Design review of the part built by this model. Coordinates are the model's own, in mm. Face numbers are marked on the shaded views. A direction names the side the tool comes from. Coordinates: 2 decimals unless noted, no trailing zeros. Write each loop counter-clockwise with the first axis right and the second up, starting at its lowest first coordinate (ties: lowest second). Pieces come first, ordered by that corner, then holes.
Q1. Add section B-B, the plane y = 8.25. Give the boundary of the cut face in (x, z), plus the area to 3 significant figures.
Q2. To check wall thickness, follow probe 1 along X at (y, z) = (8.25, 8.75); probe 2 along Y at (x, z) = (16.6, 3); probe 3 along X at (y, z) = (4.25, 10). State the ranges of each line that lie inside material, in increasing order.
Q3. Add section D-D, the plane z = 6. Give the boundary of the cut face in (x, y), plus the area to 3 significant figures.
Q4. The part is to be moulded in two halves that separate along X. For the marked faces 6, 7, 8 and 9, say which applies: +X half, -X half, draft (parallel to the pull), parting line (faces both ways), or undercut.
Q5. Add section A-A, the plane x = 16.6. Give the boundary of the cut face in (y, z).
Q6. Add section C-C, the plane z = 11.5. Give the boundary of the cut face in (x, y), plus the area to 3 significant figures.
Q7. Machinability: for the marked faces 1, 2, 3, 4 and 5, which of the approach directions +Z, -Z, +X, -X, +Y, -Y give a long, thin tool a straight path to every point of the face, cutting with its end or side? Answer none if there is none.
Q8. Clearance check with flat-ended pins moving along their axes: pin 1 Ø2.5 at (x, y) = (31.5, 16) entering from +Z; pin 2 Ø1.7 at (x, z) = (31, 9) entering from -Y; pin 3 Ø6 at (x, y) = (16.6, 6.5) entering from -Z. State where each tip first meets the part, or that it passes through.
from build123d import *

# Parameters (mm, degrees)
EXTRUDE_1_DEPTH     = 3.2
EXTRUDE_2_DEPTH     = 2.6
EXTRUDE_3_DEPTH     = 3
CUT_EXTRUDE_1_DEPTH = 2.1
SKETCH_5_R          = 2.6
CUT_EXTRUDE_2_DEPTH = 1.1
CUT_EXTRUDE_3_DEPTH = 2.1
SKETCH_7_R          = 2.6
CUT_EXTRUDE_4_DEPTH = 0.9
SKETCH_8_R          = 2
CUT_EXTRUDE_5_DEPTH = 1.8


with BuildPart() as part:
    # ｽｹｯﾁ1 → ﾎﾞｽ - 押し出し1 (new body)
    with BuildSketch(Plane.XY):
        with BuildLine():
            Line((0, 0), (13.621587752, 0))
            ThreePointArc((13.621587752, 0), (16.6, -0.649879964), (19.578412248, 0))
            Line((19.578412248, 0), (33.2, 0))
            Line((33.2, 0), (33.2, 13.000240072))
            Line((33.2, 13.000240072), (19.578412248, 13.000240072))
            ThreePointArc((19.578412248, 13.000240072), (16.6, 13.650120036), (13.621587752, 13.000240072))
            Line((13.621587752, 13.000240072), (0, 13.000240072))
            Line((0, 13.000240072), (0, 0))
        make_face()
    extrude(amount=EXTRUDE_1_DEPTH)

    # ｽｹｯﾁ2 → ﾎﾞｽ - 押し出し2 (add)
    with BuildSketch(Plane.ZY):
        with BuildLine():
            Line((3.199725342, 0), (15.472038891, 7.74466563))
            ThreePointArc((15.472038891, 7.74466563), (17.190896421, 14.371374104), (10.684882054, 16.501987504))
            Line((10.684882054, 16.501987504), (3.199725342, 13.000240072))
            Line((3.199725342, 13.000240072), (3.199725342, 0))
        make_face()
    extrude(amount=-EXTRUDE_2_DEPTH)

    # ｽｹｯﾁ3 → ﾎﾞｽ - 押し出し3 (add)
    with BuildSketch(Plane(origin=(33.2, 0, 0), x_dir=(0, 0, -1), z_dir=(1, 0, 0))):
        with BuildLine():
            Line((-3.199725342, 13.000240072), (-8.051923005, 17.315733546))
            ThreePointArc((-8.051923005, 17.315733546), (-18.828777882, 15.822754082), (-15.654913036, 5.416209475))
            Line((-15.654913036, 5.416209475), (-3.199725342, 0))
            Line((-3.199725342, 0), (-3.199725342, 13.000240072))
        make_face()
    extrude(amount=-EXTRUDE_3_DEPTH)

    # ｽｹｯﾁ4 → ｶｯﾄ - 押し出し1 (cut)
    with BuildSketch(Plane(origin=(0, 0, 0), x_dir=(-1, 0, 0), z_dir=(0, 0, -1))):
        with BuildLine():
            Line((-19.223176421, 11.277459888), (-19.223176421, 9.123296456))
            Line((-19.223176421, 9.123296456), (-21.377339853, 9.123296456))
            ThreePointArc((-21.377339853, 9.123296456), (-22.05014042, 6.500120036), (-21.377339853, 3.876943615))
            Line((-21.377339853, 3.876943615), (-19.223176421, 3.876943615))
            Line((-19.223176421, 3.876943615), (-19.223176421, 1.722780183))
            ThreePointArc((-19.223176421, 1.722780183), (-16.6, 1.049979616), (-13.976823579, 1.722780183))
            Line((-13.976823579, 1.722780183), (-13.976823579, 3.876943615))
            Line((-13.976823579, 3.876943615), (-11.822660147, 3.876943615))
            ThreePointArc((-11.822660147, 3.876943615), (-11.14985958, 6.500120036), (-11.822660147, 9.123296456))
            Line((-11.822660147, 9.123296456), (-13.976823579, 9.123296456))
            Line((-13.976823579, 9.123296456), (-13.976823579, 11.277459888))
            ThreePointArc((-13.976823579, 11.277459888), (-16.6, 11.950260456), (-19.223176421, 11.277459888))
        make_face()
    extrude(amount=-CUT_EXTRUDE_1_DEPTH, mode=Mode.SUBTRACT)

    # ｽｹｯﾁ5 → ｶｯﾄ - 押し出し2 (cut)
    with BuildSketch(Plane(origin=(0, 0, 2.1), x_dir=(-1, 0, 0), z_dir=(0, 0, -1))):
        with Locations((-16.6, 6.500120036)):
            Circle(SKETCH_5_R)
    extrude(amount=-CUT_EXTRUDE_2_DEPTH, mode=Mode.SUBTRACT)

    # ｽｹｯﾁ6 → ｶｯﾄ - 押し出し3 (cut)
    with BuildSketch(Plane.ZY.offset(-30.2)):
        with BuildLine():
            Line((15.503618238, 7.124116138), (15.503618238, 9.2730851))
            Line((15.503618238, 9.2730851), (17.6525872, 9.2730851))
            ThreePointArc((17.6525872, 9.2730851), (18.353618238, 11.9730851), (17.6525872, 14.6730851))
            Line((17.6525872, 14.6730851), (15.503618238, 14.6730851))
            Line((15.503618238, 14.6730851), (15.503618238, 16.822054063))
            ThreePointArc((15.503618238, 16.822054063), (12.803618238, 17.5230851), (10.103618238, 16.822054063))
            Line((10.103618238, 16.822054063), (10.103618238, 14.6730851))
            Line((10.103618238, 14.6730851), (7.954649275, 14.6730851))
            ThreePointArc((7.954649275, 14.6730851), (7.253618238, 11.9730851), (7.954649275, 9.2730851))
            Line((7.954649275, 9.2730851), (10.103618238, 9.2730851))
            Line((10.103618238, 9.2730851), (10.103618238, 7.124116138))
            ThreePointArc((10.103618238, 7.124116138), (12.803618238, 6.4230851), (15.503618238, 7.124116138))
        make_face()
    extrude(amount=-CUT_EXTRUDE_3_DEPTH, mode=Mode.SUBTRACT)

    # ｽｹｯﾁ7 → ｶｯﾄ - 押し出し4 (cut)
    with BuildSketch(Plane.ZY.offset(-32.3)):
        with Locations((12.803618238, 11.9730851)):
            Circle(SKETCH_7_R)
    extrude(amount=-CUT_EXTRUDE_4_DEPTH, mode=Mode.SUBTRACT)

    # ｽｹｯﾁ8 → ｶｯﾄ - 押し出し5 (cut)
    with BuildSketch(Plane(origin=(2.6, 0, 0), x_dir=(0, 0, -1), z_dir=(1, 0, 0))):
        with Locations((-12.803618238, 11.9730851)):
            Circle(SKETCH_8_R)
    extrude(amount=-CUT_EXTRUDE_5_DEPTH, mode=Mode.SUBTRACT)


solid = part.part
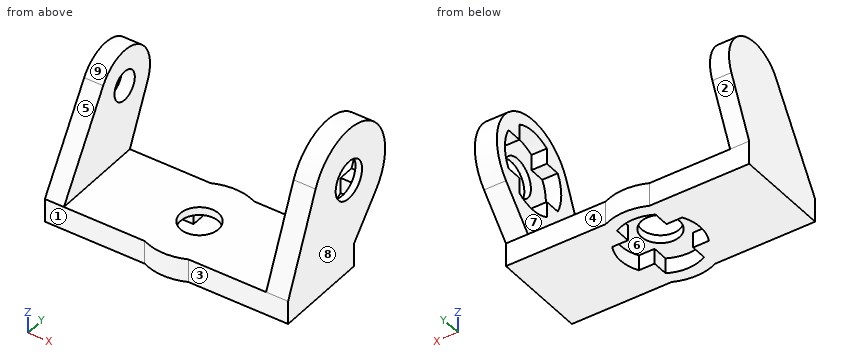
Here are the results:
1. outline: (0, 0) - (11.44, 0) - (11.44, 2.1) - (14.68, 2.1) - (14.68, 3.2) - (2.6, 3.2) - (2.6, 16.14) - (0, 16.14) - close; (18.52, 2.1) - (21.76, 2.1) - (21.76, 0) - (33.2, 0) - (33.2, 18.91) - (30.2, 18.91) - (30.2, 15.5) - (32.3, 15.5) - (32.3, 10.1) - (30.2, 10.1) - (30.2, 3.2) - (18.52, 3.2) - close
1. area: 150 mm2
2. probe 1: x = 0 to 2.6, 30.2 to 33.2
2. probe 2: y = -0.65 to 3.9, 9.1 to 13.65
2. probe 3: x = 30.2 to 33.2
3. outline: (0, 1.77) - (2.6, 1.77) - (2.6, 14.31) - (0, 14.31) - close; (30.2, 1.22) - (33.2, 1.22) - (33.2, 15.49) - (30.2, 15.49) - close
3. area: 75.4 mm2
4. face 6: undercut
4. face 7: undercut
4. face 8: +X half
4. face 9: draft
5. outline: (-0.65, 0) - (1.05, 0) - (1.05, 2.1) - (3.9, 2.1) - (3.9, 3.2) - (-0.65, 3.2) - close; (9.1, 2.1) - (11.95, 2.1) - (11.95, 0) - (13.65, 0) - (13.65, 3.2) - (9.1, 3.2) - close
6. outline: (0, 5.24) - (2.6, 5.24) - (2.6, 10.46) - (0.8, 10.46) - (0.8, 13.49) - (2.6, 13.49) - (2.6, 16.8) - (0, 16.8) - close; (30.2, 3.61) - (33.2, 3.61) - (33.2, 9.72) - (32.3, 9.72) - (32.3, 6.58) - (30.2, 6.58) - close; (30.2, 17.37) - (32.3, 17.37) - (32.3, 14.22) - (33.2, 14.22) - (33.2, 19) - (30.2, 19) - close
6. area: 44.1 mm2
7. face 1: +Z, -Z, -X, -Y
7. face 2: -Z, -X, +Y
7. face 3: +Z, -Z, +X, -Y
7. face 4: -Z, +X, +Y
7. face 5: +Z, -X, -Y
8. pin 1: stops at z = 19.39
8. pin 2: stops at y = 2.15
8. pin 3: stops at z = 2.1
